from build123d import *

# Parameters (mm, degrees)
SZKIC1_R                    = 3.5
SZKIC1_R_2                  = 1.5
DODANIE_WYCI_GNI_CIE1_DEPTH = 2


with BuildPart() as part:
    # Szkic1 → Dodanie-wyciągnięcie1 (new body)
    with BuildSketch(Plane.XY):
        with BuildLine():
            Line((0, 0), (0, 28))
            Line((0, 28), (26, 28))
            Line((26, 28), (26, 21.080196399))
            ThreePointArc((26, 21.080196399), (23.68869542, 14), (26, 6.919803601))
            Line((26, 6.919803601), (26, 0))
            Line((26, 0), (0, 0))
        make_face()
        with Locations((17.18869542, 14)):
            Circle(SZKIC1_R, mode=Mode.SUBTRACT)
        with Locations((17, 5)):
            Circle(SZKIC1_R_2, mode=Mode.SUBTRACT)
        with Locations((5, 5)):
            Circle(SZKIC1_R_2, mode=Mode.SUBTRACT)
        with Locations(Location((17, 23, 0), (0, 0, 180))):
            Circle(SZKIC1_R_2, mode=Mode.SUBTRACT)
        with Locations(Location((5, 23, 0), (0, 0, 180))):
            Circle(SZKIC1_R_2, mode=Mode.SUBTRACT)
    extrude(amount=DODANIE_WYCI_GNI_CIE1_DEPTH)


solid = part.part
Input: part model. Units: mm. Frame: model coordinates. Coordinates: 2 decimals unless noted, no trailing zeros. Order: outer loops, then holes, each group sorted by start corner. A loop starts at its lowest first (then second) coordinate and runs counter-clockwise, first axis right, second up. Notation, with made-up numbers: M 84.25,14.25 L 137.25,14.25 A24 ccw 137.25,31.25 Z; hole C 36.5,0.25 d1. An arc over 180 degrees is marked long. Answer in a Markdown table with one row per item.
(1) Section query C-C, the plane z = 1.65. Output: boundary loops of the cut face in (x, y), plus the area to 3 significant figures.
Numbers:
| item | result |
|---|---|
| outline | M 0,0 L 26,0 L 26,6.92 A12 cw 26,21.08 L 26,28 L 0,28 Z; hole C 5,5 d3; hole C 5,23 d3; hole C 17.19,14 d7; hole C 17,5 d3; hole C 17,23 d3 |
| area | 639 mm^2 |
(2) Section query B-B, the plane x = 5. Output: boundary loops of the cut face in (y, z), plus the area to 3 significant figures.
Numbers:
| item | result |
|---|---|
| outline | M 0,0 L 3.5,0 L 3.5,2 L 0,2 Z; M 6.5,0 L 21.5,0 L 21.5,2 L 6.5,2 Z; M 24.5,0 L 28,0 L 28,2 L 24.5,2 Z |
| area | 44.0 mm^2 |
(3) Section query A-A, the plane y = 14. Output: boundary loops of the cut face in (x, z), plus the area to 3 significant figures.
Numbers:
| item | result |
|---|---|
| outline | M 0,0 L 13.69,0 L 13.69,2 L 0,2 Z; M 20.69,0 L 23.69,0 L 23.69,2 L 20.69,2 Z |
| area | 33.4 mm^2 |
(4) Section query D-D, the plane y = 5. Output: boundary loops of the cut face in (x, z).
Numbers:
| item | result |
|---|---|
| outline | M 0,0 L 3.5,0 L 3.5,2 L 0,2 Z; M 6.5,0 L 15.5,0 L 15.5,2 L 6.5,2 Z; M 18.5,0 L 26,0 L 26,2 L 18.5,2 Z |
(5) Material intervals for line 1 (Y direction, x = 17, z = 1.2); line 2 (X direction, y = 23, z = 1.4); line 3 (Y direction, x = 5, z = 1.1), sorted ascending. Write a range as [from, to].
Numbers:
| item | result |
|---|---|
| line 1 | y = [0, 3.5], [6.5, 10.51], [17.49, 21.5], [24.5, 28] |
| line 2 | x = [0, 3.5], [6.5, 15.5], [18.5, 26] |
| line 3 | y = [0, 3.5], [6.5, 21.5], [24.5, 28] |
(6) Draft query along X for faces 1 (the cylindrical face through (15.5, 5.07, 0.99)), 2 (the cylindrical face through (18.11, 21.99, 0.99)), 3 (the flat face through (0, 14, 1)), 4 (the flat face through (26, 25, 1)). Return one class per face: pulls with the +X half, pulls with the -X half, needs draft (parallel to the pull), parting line crosses it, or undercut.
Numbers:
| item | result |
|---|---|
| face 1 | undercut |
| face 2 | undercut |
| face 3 | pulls with the -X half |
| face 4 | pulls with the +X half |
